```python
from build123d import *

# Parameters (mm, degrees)
CROQUIS2_W              = 240
CROQUIS2_H              = 150
CROQUIS2_R              = 10
CROQUIS2_R_2            = 15
SALIENTE_EXTRUIR2_DEPTH = 10
CORTAR_EXTRUIR1_DEPTH   = 240
CORTAR_EXTRUIR2_DEPTH   = 240


with BuildPart() as part:
    # Croquis2 → Saliente-Extruir2 (new body)
    with BuildSketch(Plane.XY):
        with Locations((120, 75)):
            Rectangle(CROQUIS2_W, CROQUIS2_H)
        with Locations((60, 70)):
            Circle(CROQUIS2_R, mode=Mode.SUBTRACT)
        with Locations((180, 35)):
            Circle(CROQUIS2_R_2, mode=Mode.SUBTRACT)
        with Locations((210, 70)):
            Circle(CROQUIS2_R_2, mode=Mode.SUBTRACT)
        with Locations(Location((150, 70, 0), (0, 0, 180))):
            Circle(CROQUIS2_R_2, mode=Mode.SUBTRACT)
        with Locations(Location((180, 105, 0), (0, 0, 180))):
            Circle(CROQUIS2_R_2, mode=Mode.SUBTRACT)
    extrude(amount=SALIENTE_EXTRUIR2_DEPTH)

    # Croquis4 → Cortar-Extruir1 (cut)
    with BuildSketch(Plane(origin=(240, 0, 0), x_dir=(0, 0, -1), z_dir=(1, 0, 0))):
        Polygon((-0.025530109, 4.943381022), (-1.679665648, 0), (0, 0), align=None)
    extrude(amount=-CORTAR_EXTRUIR1_DEPTH, mode=Mode.SUBTRACT)

    # Croquis6 → Cortar-Extruir2 (cut)
    with BuildSketch(Plane(origin=(240, 0, 0), x_dir=(0, 0, -1), z_dir=(1, 0, 0))):
        Polygon((-0.025530109, 4.943381022), (0, 4.934838233), (0, -0.070345502), (-0.012765054, -0.070345502), align=None)
    extrude(amount=-CORTAR_EXTRUIR2_DEPTH, mode=Mode.SUBTRACT)


solid = part.part
```
Geometry check sheet. Reference: the model listing, model coordinates, mm. Coordinates: 2 decimals unless noted, no trailing zeros. Order: outer loops, then holes, each group sorted by start corner. A loop starts at its lowest first (then second) coordinate and runs counter-clockwise, first axis right, second up. Notation, with made-up numbers: (26.5, 23.25) - (31.5, 23.25) arc R4 cw to (31.5, 30.25) - close; hole circle Ø6 at (-16, -15.5). An arc over 180 degrees is marked (long way). Answer as a JSON object with one key per item and string values. Group by question number.
Item 1: Sectioned sample at B-B, the plane x = 180. Give the number of separate pieces and of enclosed holes in the cut face, and give its area (3 significant figures).
Item 2: Scan lines: probe 1 along Y at (x, z) = (180, 7); probe 2 along X at (y, z) = (105, 4.5); probe 3 along Y at (x, z) = (150, 3). Record each from-to range of solid material in increasing order.
Item 3: Depth check by flat-ended pin: pin 1 Ø6 at (x, y) = (91.5, 79.5) entering from -Z. Enter the tip coordinate at first touch or a pass-through.
Item 4: Draft check along Y on faces 1 (the face through (240, 74, 5)), 2 (the face through (121.68, 2.51, 0.84)), 3 (the face through (153.252, 84.643, 4.93)), 4 (the face through (118, 150, 5)). Enter one of: +Y half, -Y half, draft (parallel to the pull), parting line (faces both ways), or undercut.
Item 5: Sectioned sample at D-D, the plane z = 4. Record the cut outline in (x, y).
Item 6: Sectioned sample at A-A, the plane y = 105. Record the cut outline in (x, z), and give its area (3 significant figures).
Resolved:
{
 "1": {"separate pieces": "3", "enclosed holes": "0", "area": "896 mm^2"},
 "2": {"probe 1": "0 to 20, 50 to 90, 120 to 150", "probe 2": "0 to 165, 195 to 240", "probe 3": "0 to 55, 85 to 150"},
 "3": {"pin 1": "z = 0"},
 "4": {"face 1": "draft", "face 2": "-Y half", "face 3": "undercut", "face 4": "+Y half"},
 "5": {"outline": "(0, 0) - (240, 0) - (240, 150) - (0, 150) - close; hole circle Ø20 at (60, 70); hole circle Ø30 at (150, 70); hole circle Ø30 at (180, 35); hole circle Ø30 at (180, 105); hole circle Ø30 at (210, 70)"},
 "6": {"outline": "(0, 0) - (165, 0) - (165, 10) - (0, 10) - close; (195, 0) - (240, 0) - (240, 10) - (195, 10) - close", "area": "2,100 mm^2"}
}
